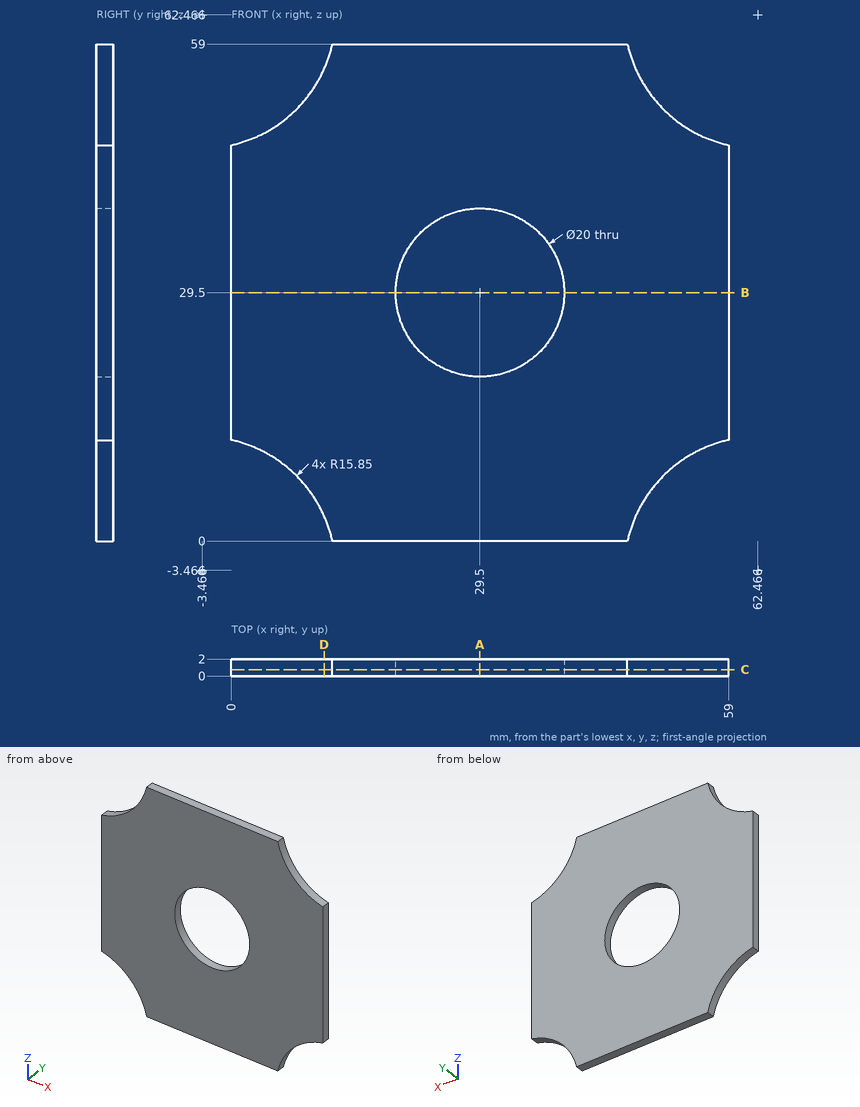
For this review, use the dimensioned drawing (mm, ordinates from the lowest corner) and the shaded views. Round coordinates to 2 decimals unless told otherwise and drop trailing zeros. Order: outer loops, then holes, each group sorted by start corner. A loop starts at its lowest first (then second) coordinate and runs counter-clockwise, first axis right, second up. Notation, with made-up numbers: (49.5, 47.25) -> (64.5, 47.25) arc R21 ccw to (64.5, 53.25) -> close; hole circle Ø3 at (-37, 86). An arc over 180 degrees is marked (long way). Put each result on its own line as item: value.
Q1. Add section B-B on z = 29.5. Write out the cut boundary in (x, y).
Check result:
outline: (0, 0) -> (19.5, 0) -> (19.5, 2) -> (0, 2) -> close; (39.5, 0) -> (59, 0) -> (59, 2) -> (39.5, 2) -> close
Q2. For probe 1 along Z at (x, y) = (29.5, 0.95); probe 2 along X at (y, z) = (0.9, 28.5), list the stretches that pass through material, from the lowest coordinate up. Write a range as [from, to].
Check result:
probe 1: [0, 19.5], [39.5, 59]
probe 2: [0, 19.55], [39.45, 59]
Q3. Add section D-D on x = 11. Write out the cut boundary in (y, z), plus the area to 3 significant figures.
Check result:
outline: (0, 3.01) -> (2, 3.01) -> (2, 55.99) -> (0, 55.99) -> close
area: 106 mm2
Q4. Add section C-C on y = 0.75. Write out the cut boundary in (x, z), plus the area to 3 significant figures.
Check result:
outline: (0, 12) arc R15.85 cw to (12, 0) -> (47, 0) arc R15.85 cw to (59, 12) -> (59, 47) arc R15.85 cw to (47, 59) -> (12, 59) arc R15.85 cw to (0, 47) -> close; hole circle Ø20 at (29.5, 29.5)
area: 2,770 mm2
Q5. Insertion check: pin 1 Ø1 at (x, y) = (10, 0) entering from +Z (1 decimal). The pin has a flat end and moves straight along its axis. Give the tip position at first contact, or say it passes through.
Check result:
pin 1: z = 55
Q6. Add section A-A on x = 29.5. Write out the cut boundary in (y, z).
Check result:
outline: (0, 0) -> (2, 0) -> (2, 19.5) -> (0, 19.5) -> close; (0, 39.5) -> (2, 39.5) -> (2, 59) -> (0, 59) -> close
